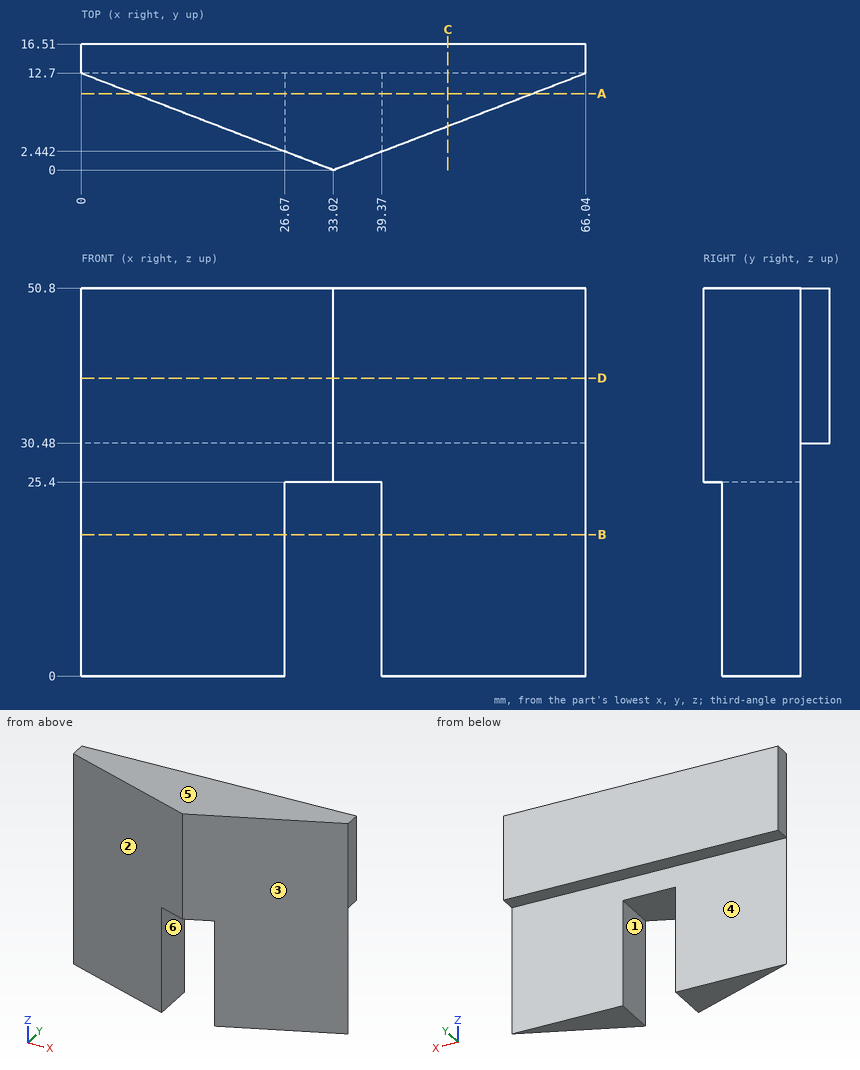
Geometry: see drawing. Coordinates: mm, zero at the bounding-box minimum. A direction names the side the tool comes from. Round coordinates to 2 decimals unless told otherwise and drop trailing zeros. Loops run counter-clockwise (first coordinate to the right, second up) from the corner with the lowest first, then second, coordinate; pieces in that order, holes last. Notation, with made-up numbers: (-10.5, 30) -> (-2.5, 30) arc R24 ccw to (-2.5, 64) -> close; hole circle Ø7 at (11, -9). An arc over 180 degrees is marked (long way). Write each question's results on one line, items separated by ' | '.
1. Section C-C (x = 48). Return loops of the section in (y, z).
Geometry results:
outline: (5.76, 0) -> (12.7, 0) -> (12.7, 30.48) -> (16.51, 30.48) -> (16.51, 50.8) -> (5.76, 50.8) -> close
2. Section D-D (z = 39). Return loops of the section in (x, y), and give its area (3 significant figures).
Geometry results:
outline: (0, 12.7) -> (33.02, 0) -> (66.04, 12.7) -> (66.04, 16.51) -> (0, 16.51) -> close | area: 671 mm2
3. Ray query, line 1 (Z direction, x = 38, y = 11); line 2 (Z direction, x = 50.5, y = 13.5); line 3 (Y direction, x = 26, z = 7.5). Return the intervals inside material, ascending. Write a range as from..to.
Geometry results:
line 1: 25.4..50.8 | line 2: 30.48..50.8 | line 3: 2.7..12.7
4. Section A-A (y = 10). Return loops of the section in (x, z), and give its area (3 significant figures).
Geometry results:
outline: (7.02, 0) -> (26.67, 0) -> (26.67, 25.4) -> (39.37, 25.4) -> (39.37, 0) -> (59.02, 0) -> (59.02, 50.8) -> (7.02, 50.8) -> close | area: 2,320 mm2
5. Set-up query: the marked faces 5 and 6. Return all of +Z, -Z, +X, -X, +Y, -Y with unobstructed straight access to the full face (end or side cutting, diameter ignored); none if empty.
Geometry results:
face 5: +Z, +X, -X, +Y, -Y | face 6: -Z, +Y, -Y
6. Mould query, pull axis X, two halves, no side actions, for the marked faces 1, 2, 3 and 4. Classes: +X half, -X half, draft (parallel to the pull), parting line (faces both ways), or undercut.
Geometry results:
face 1: undercut | face 2: -X half | face 3: +X half | face 4: draft
7. First-contact query: P1, Ø1.1, axis at x = 27, y = 14.5, coming from the -Z side; P2, Ø5, axis at x = 7.5, z = 45.5, coming from the -Y side. Flat tips, straight axial feed; report the tip coordinate or a pass-through.
Geometry results:
P1: z = 30.48 | P2: y = 8.85
8. Section B-B (z = 18.5). Return loops of the section in (x, y).
Geometry results:
outline: (0, 12.7) -> (26.67, 2.44) -> (26.67, 12.7) -> close; (39.37, 2.44) -> (66.04, 12.7) -> (39.37, 12.7) -> close
